```python
from build123d import *

# Parameters (mm, degrees)
BOSS_EXTRUDE1_START = -34.5
SKETCH2_W           = 34.4
SKETCH2_H           = 20.4
SKETCH2_R           = 1.25
BOSS_EXTRUDE1_DEPTH = 3
SKETCH1_W           = 13
SKETCH1_H           = 3
BOSS_EXTRUDE2_DEPTH = 20.4
SKETCH1_3_W         = 20
SKETCH1_3_H         = 34.4
SKETCH1_3_W_2       = 10
SKETCH1_3_H_2       = 3
SKETCH1_3_W_3       = 3
BOSS_EXTRUDE3_DEPTH = 3
SKETCH1_4_W         = 3
SKETCH1_4_H         = 34.4
SKETCH1_4_W_2       = 10
SKETCH1_4_H_2       = 3
SKETCH1_4_W_3       = 20
BOSS_EXTRUDE4_DEPTH = 100
SKETCH4_W           = 12
SKETCH4_H           = 10
CUT_EXTRUDE1_DEPTH  = 132
SKETCH7_W           = 50
SKETCH7_H           = 57
SKETCH7_R           = 2.125
BOSS_EXTRUDE5_DEPTH = 7.5


with BuildPart() as part:
    # Sketch2 → Boss-Extrude1 (new body)
    with BuildSketch(Plane(origin=(0, 0, 0), x_dir=(0, 0, -1), z_dir=(1, 0, 0)).offset(BOSS_EXTRUDE1_START)):
        with Locations((0, 10.2)):
            Rectangle(SKETCH2_W, SKETCH2_H)
        with Locations((-14.8, 18)):
            Circle(SKETCH2_R, mode=Mode.SUBTRACT)
        with Locations(Location((-14.8, 2, 0), (0, 0, 180))):
            Circle(SKETCH2_R, mode=Mode.SUBTRACT)
        with Locations((15.2, 2)):
            Circle(SKETCH2_R, mode=Mode.SUBTRACT)
        with Locations(Location((15.2, 18, 0), (0, 0, 180))):
            Circle(SKETCH2_R, mode=Mode.SUBTRACT)
    extrude(amount=-BOSS_EXTRUDE1_DEPTH)

    # Sketch1 → Boss-Extrude2 (add)
    with BuildSketch(Plane(origin=(0, 0, 0), x_dir=(1, 0, 0), z_dir=(0, 1, 0))):
        with Locations((-31, -18.7)):
            Rectangle(SKETCH1_W, SKETCH1_H)
        with Locations((-31, 18.7)):
            Rectangle(SKETCH1_W, SKETCH1_H)
    extrude(amount=BOSS_EXTRUDE2_DEPTH)

    # Sketch1<3> → Boss-Extrude3 (add)
    with BuildSketch(Plane(origin=(0, 0, 0), x_dir=(1, 0, 0), z_dir=(0, 1, 0))):
        with Locations((-24.5, 0)):
            Rectangle(SKETCH1_3_W, SKETCH1_3_H)
        with Locations((-19.5, -18.7)):
            Rectangle(SKETCH1_3_W_2, SKETCH1_3_H_2)
        Polygon((-24.5, -20.2), (-24.5, -17.2), (-34.5, -17.2), (-37.5, -17.2), (-37.5, -20.2), align=None)
        with Locations((-36, 0)):
            Rectangle(SKETCH1_3_W_3, SKETCH1_3_H)
        Polygon((-34.5, 17.2), (-24.5, 17.2), (-24.5, 20.2), (-37.5, 20.2), (-37.5, 17.2), align=None)
        with Locations((-19.5, 18.7)):
            Rectangle(SKETCH1_3_W_2, SKETCH1_3_H_2)
    extrude(amount=-BOSS_EXTRUDE3_DEPTH)

    # Sketch1<4> → Boss-Extrude4 (add)
    with BuildSketch(Plane(origin=(0, 0, 0), x_dir=(1, 0, 0), z_dir=(0, 1, 0))):
        with Locations((-36, 0)):
            Rectangle(SKETCH1_4_W, SKETCH1_4_H)
        Polygon((-24.5, -20.2), (-24.5, -17.2), (-34.5, -17.2), (-37.5, -17.2), (-37.5, -20.2), align=None)
        with Locations((-19.5, -18.7)):
            Rectangle(SKETCH1_4_W_2, SKETCH1_4_H_2)
        with Locations((-24.5, 0)):
            Rectangle(SKETCH1_4_W_3, SKETCH1_4_H)
        Polygon((-34.5, 17.2), (-24.5, 17.2), (-24.5, 20.2), (-37.5, 20.2), (-37.5, 17.2), align=None)
        with Locations((-19.5, 18.7)):
            Rectangle(SKETCH1_4_W_2, SKETCH1_4_H_2)
    extrude(amount=-BOSS_EXTRUDE4_DEPTH)

    # Sketch4 → Cut-Extrude1 (cut)
    with BuildSketch(Plane(origin=(-34.5, 0, 0), x_dir=(0, 0, -1), z_dir=(1, 0, 0))):
        with Locations((0, 20.4)):
            Rectangle(SKETCH4_W, SKETCH4_H)
    extrude(amount=-CUT_EXTRUDE1_DEPTH, mode=Mode.SUBTRACT)


with BuildPart() as body_2:
    # Mirror6: mirrored copy
    add(part.part.mirror(Plane(origin=(0, 0, 0), x_dir=(0, 0, 1), z_dir=(1, 0, 0))))


with BuildPart() as part_1:
    add(part.part)

    add(body_2.part)  # Boss-Extrude5 merges body 2
    # Sketch7 → Boss-Extrude5 (add)
    # profile 1 of 2: a face of its own
    with BuildSketch(Plane.XZ.offset(100)):
        Polygon((-14.5, -20.2), (14.5, -20.2), (37.5, -20.2), (37.5, -40.2), (-37.5, -40.2), (-37.5, -20.2), align=None)
        with BuildLine():
            ThreePointArc((-15, -28.5), (-18, -25.5), (-21, -28.5))
            Line((-21, -28.5), (-21, -32.5))
            ThreePointArc((-21, -32.5), (-18, -35.5), (-15, -32.5))
            Line((-15, -32.5), (-15, -28.5))
        make_face(mode=Mode.SUBTRACT)
        with BuildLine():
            ThreePointArc((21, -28.5), (18, -25.5), (15, -28.5))
            Line((15, -28.5), (15, -32.5))
            ThreePointArc((15, -32.5), (18, -35.5), (21, -32.5))
            Line((21, -32.5), (21, -28.5))
        make_face(mode=Mode.SUBTRACT)
    # profile 2 of 2: a face of its own
    with BuildSketch(Plane.XZ.offset(100)):
        with Locations((0, -68.7)):
            Rectangle(SKETCH7_W, SKETCH7_H)
        with Locations(Location((-21.035, -92.99, 0), (0, 0, 270))):
            Circle(SKETCH7_R, mode=Mode.SUBTRACT)
        with Locations(Location((21.035, -92.99, 0), (0, 0, 270))):
            Circle(SKETCH7_R, mode=Mode.SUBTRACT)
        with Locations(Location((-21.035, -44.95, 0), (0, 0, 270))):
            Circle(SKETCH7_R, mode=Mode.SUBTRACT)
        with Locations(Location((21.035, -44.95, 0), (0, 0, 270))):
            Circle(SKETCH7_R, mode=Mode.SUBTRACT)
    extrude(amount=-BOSS_EXTRUDE5_DEPTH)


solid = part_1.part
```
The model under review builds one solid part; all positions refer to its coordinate system, in mm. A direction names the side the tool comes from. Round coordinates to 2 decimals unless told otherwise and drop trailing zeros. Loops run counter-clockwise (first coordinate to the right, second up) from the corner with the lowest first, then second, coordinate; pieces in that order, holes last. Notation, with made-up numbers: M 8.25,59 L 19.25,59 A19 cw 19.25,67 Z; hole C -16,68 d8. An arc over 180 degrees is marked long. Write item = value, one per line.
Item 1: Take a section at C-C on x = 31.5. Write out the cut boundary in (y, z).
Return value:
outline = M -100,-40.2 L -92.5,-40.2 L -92.5,-20.2 L 20.4,-20.2 L 20.4,-17.2 L 0,-17.2 L 0,17.2 L 20.4,17.2 L 20.4,20.2 L -100,20.2 Z
Item 2: The part is to be moulded in two halves that separate along X. For faces 4 (the flat face through (25, -96, -69)), 5 (the flat face through (24.5, 10, -19)), 6 (the flat face through (-26, -35, -20.2)), say which applies: released by +X, released by -X, zero draft, split by the parting line, or undercut.
Return value:
face_4 = released by +X
face_5 = undercut
face_6 = zero draft
Item 3: Take a section at B-B on y = -49. Write out the cut boundary in (x, z).
Return value:
outline = M -37.5,-20.2 L -14.5,-20.2 L -14.5,20.2 L -37.5,20.2 Z; M 14.5,-20.2 L 37.5,-20.2 L 37.5,20.2 L 14.5,20.2 Z
Item 4: For line 1 (X direction, y = -97.75, z = -92.99); line 2 (Y direction, x = -35.55, z = -15.2); line 3 (X direction, y = -12, z = 10), list the stretches that pass through material, from the lowest coordinate up. Write a range as [from, to].
Return value:
line_1 = [-25, -23.16], [-18.91, 18.91], [23.16, 25]
line_2 = [-100, 0.75], [3.25, 16.75], [19.25, 20.4]
line_3 = [-37.5, -14.5], [14.5, 37.5]
Item 5: Insertion check: P1, Ø2.5, axis at x = -36, y = 16.5, coming from the -Z side; P2, Ø1.5, axis at x = 7.5, z = -67.5, coming from the +Y side; P3, Ø1.5, axis at y = 2, z = -15.2, coming from the -X side; P4, Ø8, axis at y = -97, z = -57.5, coming from the +X side. Each pin has a flat end and moves straight along its axis. Give the tip position at first contact, or say it passes through.
Return value:
P1 = -20.2
P2 = -92.5
P3 = through
P4 = 25
Item 6: Take a section at A-A on z = -7.5. Write out the cut boundary in (x, y), then the cut area to 3 significant figures.
Return value:
outline = M -37.5,-100 L -14.5,-100 L -14.5,0 L -34.5,0 L -34.5,20.4 L -37.5,20.4 Z; M 14.5,-100 L 37.5,-100 L 37.5,20.4 L 34.5,20.4 L 34.5,0 L 14.5,0 Z
area = 4,720 mm2
Item 7: Machinability: for faces 1 (the flat face through (-30, 10, 17.2)), 2 (the flat face through (-21, -96, -30)), 3 (the flat face through (1, -92.5, -58)), which of the approach directions +Z, -Z, +X, -X, +Y, -Y give a long, thin tool a straight path to every point of the face, cutting with its end or side? Answer none if there is none.
Return value:
face_1 = +Y
face_2 = +Y, -Y
face_3 = -Z, +X, -X, +Y
Item 8: Take a section at D-D on z = -82. Write out the cut boundary in (x, y).
Return value:
outline = M -25,-100 L 25,-100 L 25,-92.5 L -25,-92.5 Z
